The figure shows three views and two pictorial views of one solid part (mm, origin at its lowest corner). Answer the questions. Give positions to 0.01 mm unless a question says otherwise; leave off trailing zeros. Loops run counter-clockwise (first coordinate to the right, second up) from the corner with the lowest first, then second, coordinate; pieces in that order, holes last. Notation, with made-up numbers: M 14.25,-5 L 57.25,-5 A20 cw 57.25,17 Z; hole C 39,77.5 d1. An arc over 180 degrees is marked long. Answer as a JSON object with one key per item and string values. Group by question number.
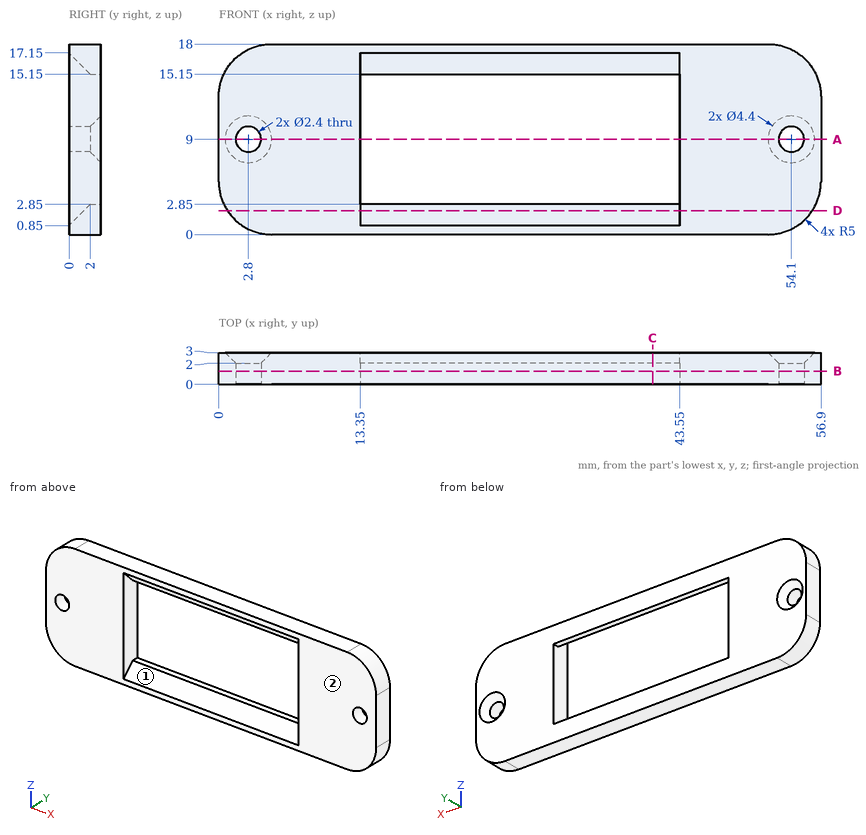
Item 1: A cutting plane is placed at D-D (z = 2.25). Determine the outline of the cut face in (x, y).
Item 2: A cutting plane is placed at C-C (x = 41). Determine the outline of the cut face in (y, z).
Item 3: For a pull along X with two mould halves and no side action, classify the marked faces 1 and 2 as pulls with the +X half, pulls with the -X half, needs draft (parallel to the pull), parting line crosses it, or undercut.
Item 4: A cutting plane is placed at B-B (y = 1.25). Determine the outline of the cut face in (x, z).
Item 5: A cutting plane is placed at A-A (z = 9). Determine the outline of the cut face in (x, y).
Item 6: Find the intervals of material crossed by probe 1 along X at (y, z) = (0.85, 9); probe 2 along X at (y, z) = (2.6, 6); probe 3 along X at (y, z) = (2.8, 7.5), in increasing order. Write a range as [from, to].
Item 7: Given pin 1 Ø1.5 at (y, z) = (1.5, 3) entering from -X, flat-ended and moving along its own axis, determine where the tip first touches the part or whether it passes through.
The answers:
{
 "1": {"outline": "M 0.82,0 L 13.35,0 L 13.35,1.4 L 43.55,1.4 L 43.55,0 L 56.08,0 L 56.08,3 L 0.82,3 Z"},
 "2": {"outline": "M 0,0 L 3,0 L 3,2.85 L 2,2.85 L 0,0.85 Z; M 0,17.15 L 2,15.15 L 3,15.15 L 3,18 L 0,18 Z"},
 "3": {"face 1": "undercut", "face 2": "needs draft"},
 "4": {"outline": "M 0,5 A5 ccw 5,0 L 51.9,0 A5 ccw 56.9,5 L 56.9,13 A5 ccw 51.9,18 L 5,18 A5 ccw 0,13 Z; hole C 2.8,9 d2.4; hole M 13.35,2.1 L 43.55,2.1 L 43.55,15.9 L 13.35,15.9 Z; hole C 54.1,9 d2.4"},
 "5": {"outline": "M 0,0 L 1.6,0 L 1.6,2 L 0.6,3 L 0,3 Z; M 4,0 L 13.35,0 L 13.35,3 L 5,3 L 4,2 Z; M 43.55,0 L 52.9,0 L 52.9,2 L 51.9,3 L 43.55,3 Z; M 55.3,0 L 56.9,0 L 56.9,3 L 56.3,3 L 55.3,2 Z"},
 "6": {"probe 1": "x = [0, 1.6], [4, 13.35], [43.55, 52.9], [55.3, 56.9]", "probe 2": "x = [0, 13.35], [43.55, 56.9]", "probe 3": "x = [0, 1.48], [4.12, 13.35], [43.55, 52.78], [55.42, 56.9]"},
 "7": {"pin 1": "stops at x = 0.16"}
}
